Geometry check sheet. Reference: the model listing, model coordinates, mm. Coordinates: 2 decimals unless noted, no trailing zeros. Write each loop counter-clockwise with the first axis right and the second up, starting at its lowest first coordinate (ties: lowest second). Pieces come first, ordered by that corner, then holes. Notation, with made-up numbers: (36, 89.25) -> (67, 89.25) arc R17 ccw to (67, 96.25) -> close; hole circle Ø7 at (49, 1). An arc over 180 degrees is marked (long way). One line per question, with ' | ' between items.
from build123d import *

# Parameters (mm, degrees)
TD_SKETCH_R                             = 0.79248
TL_FEATURE_DEPTH                        = 21.0312
TDF_STD_SKETCH_W                        = 2.09296
TDF_STD_SKETCH_H                        = 2.09296
TDF_STD_FEATURE_DEPTH                   = 22.061040395
ISA_20_STD_FEATURE_DEPTH                = 22.061040395
ISA_20_STD_FEATURE_DEPTH_BACK           = 22.061040395
F_10BA_STD_FEATURE_DEPTH                = 22.061040395
F_10BA_STD_FEATURE_DEPTH_BACK           = 22.061040395
FRO_STD_FEATURE_DEPTH                   = 22.061040395
FRO_STD_FEATURE_DEPTH_BACK              = 22.061040395
C_STD_FEATURE_DEPTH                     = 22.061040395
C_STD_FEATURE_DEPTH_BACK                = 22.061040395
ERW_STD_FEATURE_DEPTH                   = 0.0254
H_STD_FEATURE_REACH                     = 22.922
H_STD_SKETCH_R                          = 0.02286
H_STD_SKETCH_3_R                        = 0.02286
FUNNEL_FINAL_DIAMETRE_STD_FEATURE_DEPTH = 2.499995
FUNNEL_FINAL_DIAMETRE_STD_FEATURE_DRAFT = -22.5
ROUND_BR_STD_FEATURE_START              = -1
ROUND_BR_STD_FEATURE_DEPTH              = 0.96499722


with BuildPart() as part:
    # TD_sketch → TL_feature (new body)
    with BuildSketch(Plane(origin=(0, 0, 0), x_dir=(1, 0, 0), z_dir=(0, 1, 0))):
        with Locations(Location((0, 0, 0), (0, 0, 270))):
            Circle(TD_SKETCH_R)
    extrude(amount=TL_FEATURE_DEPTH)

    # TDF_STD_sketch → TDF_STD_feature (cut, through all)
    with BuildSketch(Plane(origin=(0, 0, 0), x_dir=(1, 0, 0), z_dir=(0, 1, 0))):
        with Locations((-1.4224, 0)):
            Rectangle(TDF_STD_SKETCH_W, TDF_STD_SKETCH_H)
    extrude(amount=TDF_STD_FEATURE_DEPTH, mode=Mode.SUBTRACT)

    # ISA_20_STD_sketch → ISA_20_STD_feature (cut, two sides: drawn at the far end of the back side and taken through both)
    with BuildSketch(Plane(origin=(0, 0, 0), x_dir=(0, 0, -1), z_dir=(1, 0, 0)).offset(-ISA_20_STD_FEATURE_DEPTH_BACK)):
        Polygon((-12.968809457, 73.261672178), (-3.759167997, 21.0312), (-0.0508, 0), (0.0508, 0), (3.759167997, 21.0312), (12.968809457, 73.261672178), (12.968809457, -32.810750623), (-12.968809457, -32.810750623), align=None)
    extrude(amount=ISA_20_STD_FEATURE_DEPTH + ISA_20_STD_FEATURE_DEPTH_BACK, mode=Mode.SUBTRACT)

    # 10BA_STD_sketch → 10BA_STD_feature (cut, two sides: drawn at the far end of the back side and taken through both)
    with BuildSketch(Plane.XY.offset(-F_10BA_STD_FEATURE_DEPTH_BACK)):
        Polygon((-53.216424634, 0), (-0.37592, 0), (-0.27432, 0), (-0.013865644, 0.036604473), (3.688047997, 21.0312), (12.863705333, 73.068938636), (91.245889802, 2.18375769), (25.165759835, -70.885180946), align=None)
    extrude(amount=F_10BA_STD_FEATURE_DEPTH + F_10BA_STD_FEATURE_DEPTH_BACK, mode=Mode.SUBTRACT)

    # FRO_STD_sketch → FRO_STD_feature (cut, two sides: drawn at the far end of the back side and taken through both)
    with BuildSketch(Plane.XY.offset(-FRO_STD_FEATURE_DEPTH_BACK)):
        with BuildLine():
            Line((-0.37592, 52.149873762), (-0.37592, 0.0254))
            ThreePointArc((-0.37592, 0.0254), (-0.368480512, 0.007439488), (-0.35052, 0))
            Line((-0.35052, 0), (51.773953762, 0))
            Line((51.773953762, 0), (-21.941183964, -73.715137726))
            Line((-21.941183964, -73.715137726), (-74.091057726, -21.565263964))
            Line((-74.091057726, -21.565263964), (-0.37592, 52.149873762))
        make_face()
    extrude(amount=FRO_STD_FEATURE_DEPTH + FRO_STD_FEATURE_DEPTH_BACK, mode=Mode.SUBTRACT)

    # C_STD_sketch → C_STD_feature (cut, two sides: drawn at the far end of the back side and taken through both)
    with BuildSketch(Plane(origin=(0, 0, 0), x_dir=(0, 0, -1), z_dir=(1, 0, 0)).offset(-C_STD_FEATURE_DEPTH_BACK)):
        with BuildLine():
            Line((-51.498419713, -8.177529753), (-0.048243287, 0))
            ThreePointArc((-0.048243287, 0), (0, 0.00381), (0.048243287, 0))
            Line((0.048243287, 0), (51.498419713, -8.177529753))
            Line((51.498419713, -8.177529753), (51.498419713, -112.369518834))
            Line((51.498419713, -112.369518834), (-51.498419713, -112.369518834))
            Line((-51.498419713, -112.369518834), (-51.498419713, -8.177529753))
        make_face()
    extrude(amount=C_STD_FEATURE_DEPTH + C_STD_FEATURE_DEPTH_BACK, mode=Mode.SUBTRACT)


with BuildPart() as body_2:
    # ERW_STD_sketch → ERW_STD_feature (new, symmetric)
    with BuildSketch(Plane.XY):
        Polygon((-0.145800064, 0.06604), (-0.145800064, 0), (-0.310900064, 0), (-0.261135355, 0.06604), align=None)
    extrude(amount=ERW_STD_FEATURE_DEPTH, both=True)

    # H_STD_sketch → H_STD_feature (add, up to next)
    with BuildSketch(Plane(origin=(-0.017961309, 0.13984774, 0), x_dir=(0, 0, -1), z_dir=(0.8660254037844415, 0.4999999999999953, 0)), mode=Mode.PRIVATE) as h_std_feature_sk1:
        with Locations(Location((0, 0, 0), (0, 0, 90))):
            Circle(H_STD_SKETCH_R)
    h_std_feature_tool1 = extrude(h_std_feature_sk1.sketch, amount=-H_STD_FEATURE_REACH, mode=Mode.PRIVATE) - body_2.part
    add(h_std_feature_tool1.solids().sort_by_distance((-0.017961, 0.139848, 0))[0])


with BuildPart() as funnel_final_diametre_std_feature_tool:
    # H_STD_sketch<3> → funnel_final_diametre_STD_feature (with draft: the straight prism first)
    with BuildSketch(Plane(origin=(-0.017961309, 0.13984774, 0), x_dir=(0, 0, -1), z_dir=(0.8660254037844415, 0.4999999999999953, 0))):
        with Locations(Location((0, 0, 0), (0, 0, 90))):
            Circle(H_STD_SKETCH_3_R)
    extrude(amount=FUNNEL_FINAL_DIAMETRE_STD_FEATURE_DEPTH)
    # funnel_final_diametre_STD_feature: the draft: its side faces are tilted about the plane it starts from
    funnel_final_diametre_std_feature_sides = [funnel_final_diametre_std_feature_tool.faces().sort_by_distance(p)[0] for p in [
        (1.075998281, 0.745049149, 0),
    ]]
    draft(funnel_final_diametre_std_feature_sides, Plane(origin=(-0.017961309, 0.13984774, 0), x_dir=(0, 0, -1), z_dir=(0.8660254037844415, 0.4999999999999953, 0)), FUNNEL_FINAL_DIAMETRE_STD_FEATURE_DRAFT)


with BuildPart() as body_2_1:
    add(body_2.part)

    # funnel_final_diametre_STD_feature: add funnel_final_diametre_std_feature_tool
    add(funnel_final_diametre_std_feature_tool.part)

    # ROUND_BR_STD_feature: read off the stored shape, not the designer's step
    # ROUND_BR_STD_feature outline → ROUND_BR_STD_feature (cut)
    with BuildSketch(Plane(origin=(0, 0, 0), x_dir=(0.79863551004729, -0.601815023152052, 0), z_dir=(0.601815023152052, 0.79863551004729, 0)).offset(ROUND_BR_STD_FEATURE_START)):
        with BuildLine():
            Line((-0.248295831, -0.0254), (-0.222895831, -0.0254))
            ThreePointArc((-0.222895831, -0.0254), (-0.240856343, -0.017960512), (-0.248295831, 0))
            Line((-0.248295831, 0), (-0.248295831, -0.0254))
        make_face()
        with BuildLine():
            Line((-0.248295831, 0.0254), (-0.248295831, 0))
            ThreePointArc((-0.248295831, 0), (-0.240856343, 0.017960512), (-0.222895831, 0.0254))
            Line((-0.222895831, 0.0254), (-0.248295831, 0.0254))
        make_face()
    extrude(amount=ROUND_BR_STD_FEATURE_DEPTH, mode=Mode.SUBTRACT)


with BuildPart() as part_1:
    add(part.part)

    # COMBINE_STD_feature: cut body 2
    add(body_2_1.part, mode=Mode.SUBTRACT)


solid = part_1.part
1. Cross-section at A-A on y = 13.75. Record the boundary of the cut face in (x, z).
Worked answers:
outline: (-0.38, -0.7) arc R0.79 ccw (long way) to (-0.38, 0.7) -> close
2. Cross-section at B-B on y = 2.5. Record the boundary of the cut face in (x, z).
Worked answers:
outline: (-0.38, -0.49) -> (0.42, -0.49) -> (0.42, 0.49) -> (-0.38, 0.49) -> close
3. Material ranges on line 1 (X direction, y = 6.25, z = 0.05); line 2 (Z direction, x = 0.3, y = 8.25); line 3 (X direction, y = 2.5, z = -0.35), recorded low to high. Write a range as from..to.
Worked answers:
line 1: -0.38..0.79 | line 2: -0.73..0.73 | line 3: -0.38..0.42
